from build123d import *

# Parameters (mm, degrees)
BASPROSKE_W                   = 5
BASPROSKE_H                   = 24
TOOTHCUT_DEPTH                = 35.307433597
TEETHCUTS_COUNT               = 30
TEETHCUTS_ANGLE               = 348
BORSKE_R                      = 1
BORE_DEPTH                    = 50.0000508
TAGLIO_ESTRUSIONE1_DEPTH      = 35.252832836
TAGLIO_ESTRUSIONE1_DEPTH_BACK = 35.252832836


with BuildPart() as part:
    # BasProSke → Base-Revolve (revolve)
    with BuildSketch(Plane(origin=(0, 0, 0), x_dir=(1, 0, 0), z_dir=(0, 1, 0)), mode=Mode.PRIVATE) as base_revolve_sk:
        with Locations((2.5, 12)):
            Rectangle(BASPROSKE_W, BASPROSKE_H)
    revolve(base_revolve_sk.sketch.rotate(Axis((-10, 0, 0), (1, 0, 0)), 180), axis=Axis((-10, 0, 0), (1, 0, 0)))

    # TooCutSke → ToothCut (cut, through all)
    with BuildSketch(Plane(origin=(0, 0, 0), x_dir=(0, 0, -1), z_dir=(1, 0, 0))):
        with BuildLine():
            ThreePointArc((0.830875803, 20.607256523), (0, 20.624), (-0.830875803, 20.607256523))
            ThreePointArc((-0.830875803, 20.607256523), (-1.224899184, 22.331948106), (-1.948690982, 23.946240803))
            ThreePointArc((-1.948690982, 23.946240803), (0, 24.0254), (1.948690982, 23.946240803))
            ThreePointArc((1.948690982, 23.946240803), (1.224899184, 22.331948106), (0.830875803, 20.607256523))
        make_face()
    toothcut = extrude(amount=TOOTHCUT_DEPTH, mode=Mode.SUBTRACT)

    # TeethCuts: ToothCut ×30 about axis
    teethcuts_axis = Axis((-10, 0, 0), (1, 0, 0))
    for i in range(1, TEETHCUTS_COUNT):
        add(toothcut.rotate(teethcuts_axis, i * TEETHCUTS_ANGLE / (TEETHCUTS_COUNT - 1)), mode=Mode.SUBTRACT)

    # BorSke → Bore (cut, symmetric)
    with BuildSketch(Plane(origin=(0, 0, 0), x_dir=(0, 0, -1), z_dir=(1, 0, 0))):
        with Locations(Location((0, 0, 0), (0, 0, 180))):
            Circle(BORSKE_R)
    extrude(amount=BORE_DEPTH, both=True, mode=Mode.SUBTRACT)

    # Schizzo2 → Taglio-Estrusione1 (cut, two sides: drawn at the far end of the back side and taken through both)
    with BuildSketch(Plane.ZY.offset(-TAGLIO_ESTRUSIONE1_DEPTH_BACK)):
        with BuildLine():
            Line((1.532970972, 2.1), (-1.532970972, 2.1))
            ThreePointArc((-1.532970972, 2.1), (-1.177768117, -2.317943542), (2.6, 0))
            ThreePointArc((2.6, 0), (2.317943542, 1.177768117), (1.532970972, 2.1))
        make_face()
    extrude(amount=TAGLIO_ESTRUSIONE1_DEPTH + TAGLIO_ESTRUSIONE1_DEPTH_BACK, mode=Mode.SUBTRACT)


solid = part.part
Source: CAD feature listing. Evaluate the final solid. Frame: model axes, mm. A direction names the side the tool comes from. Round coordinates to 2 decimals unless told otherwise and drop trailing zeros. Loops run counter-clockwise (first coordinate to the right, second up) from the corner with the lowest first, then second, coordinate; pieces in that order, holes last. Notation, with made-up numbers: (41.25, 9) - (95.25, 9) arc R25 ccw to (95.25, 27) - close; hole circle Ø9 at (-26, 34.25). An arc over 180 degrees is marked (long way). Write item = value, one per line. Start each with the question number.
Item 1: Reachability of faces 4 (the face through (2.465, -13.792, 15.334)), 5 (the face through (2.465, 3.557, 22.091)), 6 (the face through (2.465, -1.124, -22.3)) from +Z, -Z, +X, -X, +Y, -Y: full face, straight path, thin tool, end or side. Return the list, or none.
Item 2: Material intervals for line 1 (Y direction, x = 2.05, z = 0); line 2 (Z direction, x = 3.05, y = 0); line 3 (Y direction, x = 0.6, z = 22), sorted ascending.
Item 3: First-contact query: pin 1 Ø1.5 at (x, z) = (1.5, 13) entering from +Y; pin 2 Ø2 at (x, z) = (2, -6.5) entering from +Y; pin 3 Ø3 at (x, z) = (1, 17) entering from +Y. Flat tips, straight axial feed; report the tip coordinate or a pass-through.
Item 4: Mould query, pull axis Y, two halves, no side actions, for faces 1 (the face through (2.54, -9.75, 21.93)), 2 (the face through (2.54, 9.75, -21.93)), 3 (the face through (2.465, -18.846, -8.378)). Classes: released by +Y, released by -Y, zero draft, split by the parting line, or undercut.
Item 5: Section query A-A on z = 0. Output: boundary loops of the cut face in (x, y), plus the area to 3 significant figures.
Item 6: Section query B-B on y = 12.5. Output: boundary loops of the cut face in (x, z).
Results list:
q1.face_4 = +X, -X
q1.face_5 = +Z, +X, -X
q1.face_6 = -Z, +X, -X
q2.line_1 = -20.62 to -2.6, 2.1 to 20.62
q2.line_2 = -24 to -2.6, 2.6 to 24
q2.line_3 = -9.59 to -9.07, -5.72 to -3.52, -1.18 to 1.18, 3.52 to 5.72, 9.07 to 9.59
q3.pin_1 = 20.64
q3.pin_2 = 23
q3.pin_3 = 18.22
q4.face_1 = released by -Y
q4.face_2 = released by +Y
q4.face_3 = undercut
q5.outline = (0, -20.62) - (5, -20.62) - (5, -2.6) - (0, -2.6) - close; (0, 2.1) - (5, 2.1) - (5, 20.62) - (0, 20.62) - close
q5.area = 183 mm²
q6.outline = (0, -18.96) - (5, -18.96) - (5, 18.96) - (0, 18.96) - close
